Work out the finished part from the listing and answer in its coordinate system (mm). A direction names the side the tool comes from. Give positions to 0.01 mm unless a question says otherwise; leave off trailing zeros. Loops run counter-clockwise (first coordinate to the right, second up) from the corner with the lowest first, then second, coordinate; pieces in that order, holes last. Notation, with made-up numbers: (27.5, -31.75) - (75.5, -31.75) arc R31 ccw to (75.5, -6.75) - close; hole circle Ø11 at (19.5, 40.5). An arc over 180 degrees is marked (long way). One line per item, written item: value.
from build123d import *

# Parameters (mm, degrees)
BOSS_EXTRUDE1_DEPTH      = 304.8
BOSS_EXTRUDE1_DEPTH_BACK = 304.8


with BuildPart() as part:
    # Sketch3 → Boss-Extrude1 (new, two sides: drawn at the far end of the back side and taken through both)
    with BuildSketch(Plane.XY.offset(-BOSS_EXTRUDE1_DEPTH_BACK)):
        Polygon((-50, 0), (0, 0), (0, 50), (-3, 50), (-3, 3), (-50, 3), align=None)
    extrude(amount=BOSS_EXTRUDE1_DEPTH + BOSS_EXTRUDE1_DEPTH_BACK)


solid = part.part
1. For faces 1 (the flat face through (0, 25, -4)), 2 (the flat face through (-3, 27, -4)), determine the directions among +Z, -Z, +X, -X, +Y, -Y from which every point of the face is accessible in a straight line to the end or side of a thin tool.
Output:
face 1: +Z, -Z, +X, +Y, -Y
face 2: +Z, -Z, -X, +Y
2. Section A-A (z = -232) is taken. Write down the section's boundary in (x, y), and give its area (3 significant figures).
Output:
outline: (-50, 0) - (0, 0) - (0, 50) - (-3, 50) - (-3, 3) - (-50, 3) - close
area: 291 mm²
3. Section C-C (y = 8) is taken. Write down the section's boundary in (x, z).
Output:
outline: (-3, -304.8) - (0, -304.8) - (0, 304.8) - (-3, 304.8) - close
4. Section B-B (x = -33.5) is taken. Write down the section's boundary in (y, z).
Output:
outline: (0, -304.8) - (3, -304.8) - (3, 304.8) - (0, 304.8) - close
5. Flat-ended cylindrical pins translate along their axes: pin 1 Ø4 at (y, z) = (28.5, -66) entering from -X; pin 2 Ø10 at (x, z) = (-29.5, -200.5) entering from +Y. Find the tip coordinate at first contact, or state that the pin passes through.
Output:
pin 1: stops at x = -3
pin 2: stops at y = 3
6. Find the intervals of material crossed by line 1 along Y through (x, z) = (-25, -173); line 2 along X through (y, z) = (39.5, -80), in increasing order.
Output:
line 1: y = 0 to 3
line 2: x = -3 to 0
